Here's how the part is built. I have some questions about the finished solid (model axes, mm). Face numbers are marked on the shaded views. A direction names the side the tool comes from. Coordinates: 2 decimals unless noted, no trailing zeros. Write each loop counter-clockwise with the first axis right and the second up, starting at its lowest first coordinate (ties: lowest second). Pieces come first, ordered by that corner, then holes. Notation, with made-up numbers: (-19, 28.25) -> (30, 28.25) arc R22 ccw to (30, 41.25) -> close; hole circle Ø7 at (20, 24.25). An arc over 180 degrees is marked (long way). Use a Markdown table: item, result. Add a question column.
Item 1: On a 3-axis mill with a long thin cutter (end or side, diameter ignored), from which of +Z, -Z, +X, -X, +Y, -Y can I reach the whole of each face in a straight line? I mean the marked faces 1, 2 and 3. Say none if no direction works.
Item 2: Will these pins go through, and if not, where does the flat tip stop? pin 1 Ø8 at (x, y) = (-4.5, 37.5) entering from +Z; pin 2 Ø22 at (x, y) = (28.5, 23.5) entering from +Z (3 decimals); pin 3 Ø3 at (y, z) = (126.5, -8.5) entering from +X; pin 4 Ø9.5 at (y, z) = (45, 8.5) entering from +X (3 decimals).
Item 3: Imagine slicing it at C-C, the plane z = -9. Write out the boundary of the cut face in (x, y).
Item 4: Imagine slicing it at B-B, the plane x = -7. Write out the boundary of the cut face in (y, z), and give its area (3 significant figures).
Item 5: If I drill on line 1 along X through (y, z) = (57.15, 16.25) (3 decimals); line 2 along Y through (x, z) = (12.7, 10.5); line 3 along Y through (x, z) = (10, 12), over which ranges is the centre line in solid material (lowest first)? Write a range as from..to.
Item 6: Imagine slicing it at A-A, the plane y = 6.35. Write out the boundary of the cut face in (x, z) (3 decimals).
Item 7: Imagine slicing it at D-D, the plane x = 6.5. Write out the boundary of the cut face in (y, z) (3 decimals).
```python
from build123d import *

# Parameters (mm, degrees)
BOSS_EXTRUDE1_DEPTH = 25.4
SKETCH3_W           = 50.8
SKETCH3_H           = 63.5
CUT_EXTRUDE1_DEPTH  = 3.175
SKETCH4_W           = 25.4
SKETCH4_H           = 63.5
CUT_EXTRUDE2_DEPTH  = 3.175
SKETCH5_W           = 50.8
SKETCH5_H           = 63.5
CUT_EXTRUDE3_DEPTH  = 3.175
SKETCH6_W           = 25.4
SKETCH6_H           = 63.5
CUT_EXTRUDE4_DEPTH  = 3.175
SKETCH7_W           = 101.6
SKETCH7_H           = 177.8
CUT_EXTRUDE5_DEPTH  = 298.299377732
CUT_EXTRUDE7_DEPTH  = 275.74300719
CUT_EXTRUDE6_DEPTH  = 275.74300719
CUT_EXTRUDE8_DEPTH  = 271.614582269
SKETCH11_R          = 2.5527
CUT_EXTRUDE9_DEPTH  = 259.040032264
SKETCH12_R          = 2.5527
CUT_EXTRUDE10_DEPTH = 260.254504648
BOSS_EXTRUDE2_DEPTH = 25.4
CUT_EXTRUDE11_DEPTH = 263.236499242
CUT_EXTRUDE12_DEPTH = 263.052184929
CUT_EXTRUDE13_DEPTH = 266.160848634
CUT_EXTRUDE14_DEPTH = 261.679987062
CUT_EXTRUDE15_DEPTH = 250.010650693


with BuildPart() as part:
    # Sketch1 → Boss-Extrude1 (new body)
    with BuildSketch(Plane.XY):
        Polygon((50.8, 76.2), (152.4, 76.2), (152.4, 254), (-101.6, 254), (-101.6, 76.2), (0, 76.2), (0, 0), (50.8, 0), align=None)
    extrude(amount=BOSS_EXTRUDE1_DEPTH)

    # Sketch3 → Cut-Extrude1 (cut)
    with BuildSketch(Plane.XY.offset(25.4)):
        with Locations((25.4, 31.75)):
            Rectangle(SKETCH3_W, SKETCH3_H)
    extrude(amount=-CUT_EXTRUDE1_DEPTH, mode=Mode.SUBTRACT)

    # Sketch4 → Cut-Extrude2 (cut)
    with BuildSketch(Plane.ZY):
        with Locations((12.7, 31.75)):
            Rectangle(SKETCH4_W, SKETCH4_H)
    extrude(amount=-CUT_EXTRUDE2_DEPTH, mode=Mode.SUBTRACT)

    # Sketch5 → Cut-Extrude3 (cut)
    with BuildSketch(Plane(origin=(0, 0, 0), x_dir=(-1, 0, 0), z_dir=(0, 0, -1))):
        with Locations((-25.4, 31.75)):
            Rectangle(SKETCH5_W, SKETCH5_H)
    extrude(amount=-CUT_EXTRUDE3_DEPTH, mode=Mode.SUBTRACT)

    # Sketch6 → Cut-Extrude4 (cut)
    with BuildSketch(Plane(origin=(50.8, 0, 0), x_dir=(0, 0, -1), z_dir=(1, 0, 0))):
        with Locations((-12.7, 31.75)):
            Rectangle(SKETCH6_W, SKETCH6_H)
    extrude(amount=-CUT_EXTRUDE4_DEPTH, mode=Mode.SUBTRACT)

    # Sketch7 → Cut-Extrude5 (cut, through all)
    with BuildSketch(Plane.XY.offset(25.4)):
        with Locations((101.6, 165.1)):
            Rectangle(SKETCH7_W, SKETCH7_H)
    extrude(amount=-CUT_EXTRUDE5_DEPTH, mode=Mode.SUBTRACT)

    # Sketch9 → Cut-Extrude7 (cut, through all)
    with BuildSketch(Plane.XY.offset(25.4)):
        Polygon((34.65764308, 254), (50.8, 254), (50.8, 242.697), align=None)
    extrude(amount=-CUT_EXTRUDE7_DEPTH, mode=Mode.SUBTRACT)

    # Sketch8 → Cut-Extrude6 (cut, through all)
    with BuildSketch(Plane.XY.offset(25.4)):
        Polygon((34.65764308, 254), (-101.6, 59.403918632), (-101.6, 254), align=None)
    extrude(amount=-CUT_EXTRUDE6_DEPTH, mode=Mode.SUBTRACT)

    # Sketch10 → Cut-Extrude8 (cut, through all)
    with BuildSketch(Plane.XY.offset(25.4)):
        Polygon((34.65764308, 254), (45.59768076, 246.339703148), (-84.029822158, 61.212443237), (-94.969859838, 68.872740089), align=None)
    extrude(amount=-CUT_EXTRUDE8_DEPTH, mode=Mode.SUBTRACT)

    # Sketch11 → Cut-Extrude9 (cut, through all)
    with BuildSketch(Plane.XY.offset(22.225)):
        with Locations((12.7, 57.15)):
            Circle(SKETCH11_R)
        with Locations((12.7, 44.45)):
            Circle(SKETCH11_R)
        with Locations((12.7, 31.75)):
            Circle(SKETCH11_R)
        with Locations((12.7, 19.05)):
            Circle(SKETCH11_R)
        with Locations((12.7, 6.35)):
            Circle(SKETCH11_R)
        with Locations((38.1, 44.45)):
            Circle(SKETCH11_R)
        with Locations((38.1, 31.75)):
            Circle(SKETCH11_R)
        with Locations((38.1, 19.05)):
            Circle(SKETCH11_R)
        with Locations((38.1, 6.35)):
            Circle(SKETCH11_R)
        with Locations((38.1, 57.15)):
            Circle(SKETCH11_R)
    extrude(amount=-CUT_EXTRUDE9_DEPTH, mode=Mode.SUBTRACT)

    # Sketch12 → Cut-Extrude10 (cut, through all)
    with BuildSketch(Plane.ZY.offset(-3.175)):
        with Locations(Location((12.7, 57.15, 0), (0, 0, 270))):
            Circle(SKETCH12_R)
        with Locations(Location((12.7, 44.45, 0), (0, 0, 270))):
            Circle(SKETCH12_R)
        with Locations(Location((12.7, 31.75, 0), (0, 0, 270))):
            Circle(SKETCH12_R)
        with Locations(Location((12.7, 19.05, 0), (0, 0, 270))):
            Circle(SKETCH12_R)
        with Locations(Location((12.7, 6.35, 0), (0, 0, 270))):
            Circle(SKETCH12_R)
    extrude(amount=-CUT_EXTRUDE10_DEPTH, mode=Mode.SUBTRACT)

    # Sketch17 → Boss-Extrude2 (add)
    with BuildSketch(Plane(origin=(0, 0, 0), x_dir=(-1, 0, 0), z_dir=(0, 0, -1))):
        Polygon((-45.59768076, 246.339703148), (-68.484788877, 230.313977516), (51.302461146, 59.240055162), (74.189569264, 75.265780794), align=None)
    extrude(amount=BOSS_EXTRUDE2_DEPTH)

    # Sketch18 → Cut-Extrude11 (cut, through all)
    with BuildSketch(Plane(origin=(0, 0, -25.4), x_dir=(-1, 0, 0), z_dir=(0, 0, -1))):
        Polygon((39.426979923, 76.2), (73.535421933, 76.2), (74.189569264, 75.265780794), (51.302461146, 59.240055162), align=None)
    extrude(amount=-CUT_EXTRUDE11_DEPTH, mode=Mode.SUBTRACT)

    # Sketch19 → Cut-Extrude12 (cut, through all)
    with BuildSketch(Plane.XY.offset(25.4)):
        Polygon((0, 76.2), (-43.972708631, 118.419930077), (-73.535421933, 76.2), align=None)
    extrude(amount=-CUT_EXTRUDE12_DEPTH, mode=Mode.SUBTRACT)

    # Sketch20 → Cut-Extrude13 (cut, through all)
    with BuildSketch(Plane(origin=(50.8, 0, 0), x_dir=(0, 0, -1), z_dir=(1, 0, 0))):
        Polygon((-25.4, 76.2), (-12.7, 100.289703148), (-12.7, 246.339703148), (-25.4, 246.339703148), align=None)
    extrude(amount=-CUT_EXTRUDE13_DEPTH, mode=Mode.SUBTRACT)

    # Sketch21 → Cut-Extrude14 (cut, through all)
    with BuildSketch(Plane(origin=(0, 0, -25.4), x_dir=(-1, 0, 0), z_dir=(0, 0, -1))):
        Polygon((-45.59768076, 246.339703148), (-63.283173396, 233.956187887), (28.212035852, 103.287487173), (45.897528488, 115.671002434), align=None)
    extrude(amount=-CUT_EXTRUDE14_DEPTH, mode=Mode.SUBTRACT)

    # Sketch22 → Cut-Extrude15 (cut, through all)
    with BuildSketch(Plane(origin=(0, 0, -25.4), x_dir=(-1, 0, 0), z_dir=(0, 0, -1))):
        Polygon((-50.8, 205.057481532), (-45.597680844, 208.698686951), (-63.283173396, 233.956187887), (-68.484788877, 230.313977516), align=None)
    extrude(amount=-CUT_EXTRUDE15_DEPTH, mode=Mode.SUBTRACT)


solid = part.part
```
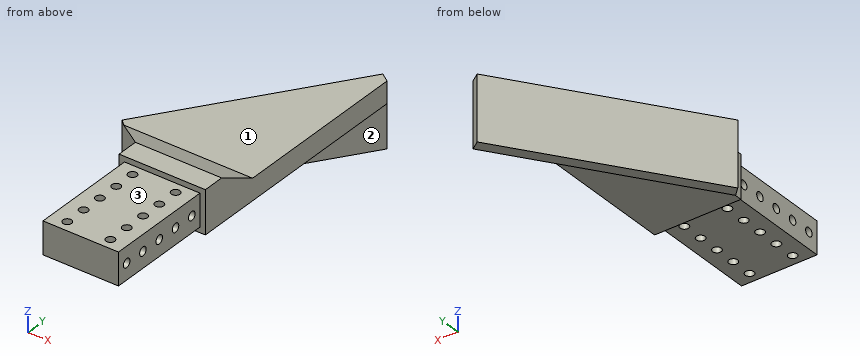
Ans:
| question | item | result |
|---|---|---|
| 1 | face 1 | +Z, +X, -X, +Y |
| 1 | face 2 | -Z, +X, -Y |
| 1 | face 3 | +Z, +X, -X, -Y |
| 2 | pin 1 | passes through |
| 2 | pin 2 | stops at z = 22.225 |
| 2 | pin 3 | stops at x = -3.16 |
| 2 | pin 4 | stops at x = 47.625 |
| 3 | outline | (-28.21, 103.29) -> (-23.58, 98.84) -> (50.8, 205.06) -> (45.6, 208.7) -> close |
| 4 | outline | (82.92, 0) -> (122.51, 0) -> (122.51, -25.4) -> (133.58, -25.4) -> (133.58, 12.7) -> (100.29, 12.7) -> (82.92, 21.86) -> close |
| 4 | area | 1,000 mm^2 |
| 5 | line 1 | x = 3.175..10.147, 15.253..35.547, 40.653..47.625 |
| 5 | line 2 | y = 0..3.8, 8.9..16.5, 21.6..29.2, 34.3..41.9, 47..54.6, 59.7..161.72 |
| 5 | line 3 | y = 0..3.9, 8.8..16.6, 21.5..29.3, 34.2..42, 46.9..54.7, 59.6..157.86 |
| 6 | outline | (3.175, 3.175) -> (10.147, 3.175) -> (10.147, 10.147) -> (3.175, 10.147) -> close; (3.175, 15.253) -> (10.147, 15.253) -> (10.147, 22.225) -> (3.175, 22.225) -> close; (15.253, 3.175) -> (35.547, 3.175) -> (35.547, 10.147) -> (15.253, 10.147) -> close; (15.253, 15.253) -> (35.547, 15.253) -> (35.547, 22.225) -> (15.253, 22.225) -> close; (40.653, 3.175) -> (47.625, 3.175) -> (47.625, 10.147) -> (40.653, 10.147) -> close; (40.653, 15.253) -> (47.625, 15.253) -> (47.625, 22.225) -> (40.653, 22.225) -> close |
| 7 | outline | (0, 3.175) -> (63.5, 3.175) -> (63.5, 0) -> (141.791, 0) -> (141.791, -25.4) -> (152.861, -25.4) -> (152.861, 12.7) -> (100.29, 12.7) -> (76.2, 25.4) -> (63.5, 25.4) -> (63.5, 22.225) -> (0, 22.225) -> close; hole circle Ø5.105 at (6.35, 12.7); hole circle Ø5.105 at (19.05, 12.7); hole circle Ø5.105 at (31.75, 12.7); hole circle Ø5.105 at (44.45, 12.7); hole circle Ø5.105 at (57.15, 12.7) |
